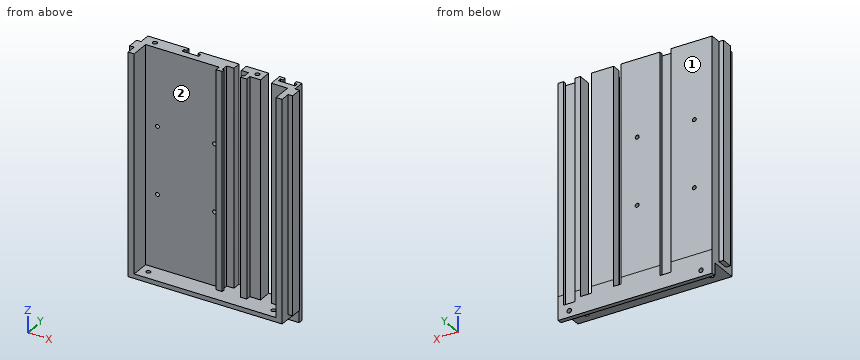
from build123d import *

# Parameters (mm, degrees)
CROQUIS1_W              = 170
CROQUIS1_H              = 50
SALIENTE_EXTRUIR1_DEPTH = 4
CROQUIS3_W              = 20
CROQUIS3_H              = 12.01
SALIENTE_EXTRUIR2_DEPTH = 194
CROQUIS22_W             = 170
CROQUIS22_H             = 21.26
CORTAR_EXTRUIR12_DEPTH  = 10
CROQUIS23_W             = 170
CROQUIS23_H             = 8.12284292
SALIENTE_EXTRUIR6_DEPTH = 11
CROQUIS25_W             = 6.514763964
CROQUIS25_H             = 194
CORTAR_EXTRUIR16_DEPTH  = 10
CROQUIS27_R             = 1.75
CORTAR_EXTRUIR17_DEPTH  = 30.74
CORTAR_EXTRUIR18_DEPTH  = 197
CROQUIS29_W             = 31.946298055
CROQUIS29_H             = 28.740140904
CORTAR_EXTRUIR19_DEPTH  = 197
CROQUIS30_R             = 2
CORTAR_EXTRUIR20_DEPTH  = 197
CROQUIS31_R             = 2
UNI_N_TECHO_DEPTH       = 10
CROQUIS33_R             = 2
CORTAR_EXTRUIR22_DEPTH  = 10
CROQUIS35_W             = 138.053701945
CROQUIS35_H             = 11
CORTAR_EXTRUIR24_DEPTH  = 4.12
SALIENTE_EXTRUIR7_DEPTH = 194


with BuildPart() as part:
    # Croquis1 → Saliente-Extruir1 (new body)
    with BuildSketch(Plane.XY):
        Rectangle(CROQUIS1_W, CROQUIS1_H)
    extrude(amount=SALIENTE_EXTRUIR1_DEPTH)

    # Croquis3 → Saliente-Extruir2 (add)
    with BuildSketch(Plane.XY.offset(4)):
        Polygon((-13.772145946, -12.69105844), (-9.772145946, -12.69105844), (-8.272145946, -12.69105844), (-8.272145946, -9.69105844), (-9.772145946, -9.69105844), (-9.772145946, -3.69105844), (9.772145946, -3.69105844), (9.772145946, -9.69105844), (8.272145946, -9.69105844), (8.272145946, -12.69105844), (9.772145946, -12.69105844), (13.772145946, -12.69105844), (13.772145946, -8.269859096), (23.357191672, -8.269859096), (23.357191672, 3.740140904), (-85, 3.740140904), (-85, -8.269859096), (-13.772145946, -8.269859096), align=None)
        with Locations((43.053701945, -2.264859096)):
            Rectangle(CROQUIS3_W, CROQUIS3_H)
    extrude(amount=SALIENTE_EXTRUIR2_DEPTH)

    # Croquis22 → Cortar-Extruir12 (cut)
    with BuildSketch(Plane(origin=(0, 0, 0), x_dir=(-1, 0, 0), z_dir=(0, 0, -1))):
        with Locations((0, 14.37)):
            Rectangle(CROQUIS22_W, CROQUIS22_H)
    extrude(amount=-CORTAR_EXTRUIR12_DEPTH, mode=Mode.SUBTRACT)

    # Croquis23 → Saliente-Extruir6 (add)
    with BuildSketch(Plane(origin=(0, 0, 0), x_dir=(-1, 0, 0), z_dir=(0, 0, -1))):
        with Locations((0, -0.32142146)):
            Rectangle(CROQUIS23_W, CROQUIS23_H)
    extrude(amount=SALIENTE_EXTRUIR6_DEPTH)

    # Croquis25 → Cortar-Extruir16 (cut)
    with BuildSketch(Plane.XZ.offset(3.69105844)):
        with Locations((0, 101)):
            Rectangle(CROQUIS25_W, CROQUIS25_H)
    extrude(amount=-CORTAR_EXTRUIR16_DEPTH, mode=Mode.SUBTRACT)

    # Croquis27 → Cortar-Extruir17 (cut)
    with BuildSketch(Plane.XZ.offset(8.269859096)):
        with Locations(Location((-69.012145946, 129.117553519, 0), (0, 0, 270))):
            Circle(CROQUIS27_R)
        with Locations(Location((-17.772145946, 129.117553519, 0), (0, 0, 270))):
            Circle(CROQUIS27_R)
        with Locations(Location((-69.012145946, 69.117553519, 0), (0, 0, 270))):
            Circle(CROQUIS27_R)
        with Locations(Location((-17.772145946, 69.117553519, 0), (0, 0, 270))):
            Circle(CROQUIS27_R)
    extrude(amount=-CORTAR_EXTRUIR17_DEPTH, mode=Mode.SUBTRACT)

    # Croquis28 → Cortar-Extruir18 (cut)
    with BuildSketch(Plane.XY.offset(198)):
        Polygon((50.605, 0.740140904), (50.605, -2.259859096), (35.605, -2.259859096), (35.605, 0.740140904), (38.105, 0.740140904), (38.105, 3.740140904), (48.105, 3.740140904), (48.105, 0.740140904), align=None)
        Polygon((-38.105, 3.740140904), (-48.105, 3.740140904), (-48.105, 0.740140904), (-50.605, 0.740140904), (-50.605, -2.259859096), (-35.605, -2.259859096), (-35.605, 0.740140904), (-38.105, 0.740140904), align=None)
    extrude(amount=-CORTAR_EXTRUIR18_DEPTH, mode=Mode.SUBTRACT)

    # Croquis29 → Cortar-Extruir19 (cut)
    with BuildSketch(Plane.XY.offset(4)):
        with Locations((69.026850973, -10.629929548)):
            Rectangle(CROQUIS29_W, CROQUIS29_H)
    extrude(amount=-CORTAR_EXTRUIR19_DEPTH, mode=Mode.SUBTRACT)

    # Croquis30 → Cortar-Extruir20 (cut)
    with BuildSketch(Plane.XY.offset(4)):
        with Locations((-72, -16.634929548)):
            Circle(CROQUIS30_R)
        with Locations((40.053701945, -16.634929548)):
            Circle(CROQUIS30_R)
    extrude(amount=-CORTAR_EXTRUIR20_DEPTH, mode=Mode.SUBTRACT)

    # Croquis31 → Unión techo (cut)
    with BuildSketch(Plane.XY.offset(198)):
        with Locations((-75, -2.264859096)):
            Circle(CROQUIS31_R)
        with Locations((16.857191672, -2.264859096)):
            Circle(CROQUIS31_R)
    extrude(amount=-UNI_N_TECHO_DEPTH, mode=Mode.SUBTRACT)

    # Croquis33 → Cortar-Extruir22 (cut)
    with BuildSketch(Plane.XZ.offset(4.38284292)):
        with Locations(Location((-75, -5.5, 0), (0, 0, 270))):
            Circle(CROQUIS33_R)
        with Locations(Location((43.053701945, -5.5, 0), (0, 0, 270))):
            Circle(CROQUIS33_R)
    extrude(amount=-CORTAR_EXTRUIR22_DEPTH, mode=Mode.SUBTRACT)

    # Croquis35 → Cortar-Extruir24 (cut)
    with BuildSketch(Plane.XZ.offset(4.38284292)):
        with Locations((-15.973149027, -5.5)):
            Rectangle(CROQUIS35_W, CROQUIS35_H)
    extrude(amount=-CORTAR_EXTRUIR24_DEPTH, mode=Mode.SUBTRACT)

    # Croquis36 → Saliente-Extruir7 (add)
    with BuildSketch(Plane.XY.offset(4)):
        Polygon((-85, -8.269859096), (-79.581388396, -8.269859096), (-79.581388396, -25), (-85, -25), (-85, -16.259859096), (-89, -16.259859096), (-89, -6.259859096), (-85, -6.259859096), align=None)
        Polygon((53.053701945, -8.269859096), (53.053701945, -6.259859096), (57.053701945, -6.259859096), (57.053701945, -16.259859096), (53.053701945, -16.259859096), (53.053701945, -25), (47.63509034, -25), (47.63509034, -8.269859096), align=None)
    extrude(amount=SALIENTE_EXTRUIR7_DEPTH)


solid = part.part
Check sheet for the modelled part. Datum: model origin and axes. Units: mm. Face numbers are marked on the shaded views. Round coordinates to 2 decimals unless told otherwise and drop trailing zeros. Order: outer loops, then holes, each group sorted by start corner. A loop starts at its lowest first (then second) coordinate and runs counter-clockwise, first axis right, second up.
(1) Draft check along X on the marked faces 1 and 2. Enter one of: pulls with the +X half, pulls with the -X half, needs draft (parallel to the pull), parting line crosses it, or undercut.
(2) Go/stop test with flat-tipped pins: P1, Ø6, axis at y = 0.5, z = 103.5, coming from the +X side; P2, Ø2, axis at x = -5.5, z = 119.5, coming from the -Y side; P3, Ø2, axis at x = 36.5, z = 145.5, coming from the -Y side. Record where each tip stops, or that it passes through.
(3) Scan lines: probe 1 along X at (y, z) = (0.25, 80.5) (3 decimals); probe 2 along X at (y, z) = (-11.5, 115); probe 3 along X at (y, z) = (-4, 157.5). Record each from-to range of solid material in increasing order.
(4) Cross-section at A-A, the plane x = -45. Enter the section's corners in (y, z), and give its area (3 significant figures).
(5) Cross-section at C-C, the plane y = -21.25. Enter the section's corners in (x, z), and give its area (3 significant figures).
(6) Cross-section at B-B, the plane z = 50. State how many separate pieces and enclosed holes the cut face has, and give its area (3 significant figures).
Check sheet entries:
1. face 1: needs draft
1. face 2: undercut
2. P1: stops at x = 53.05
2. P2: stops at y = -3.69
2. P3: stops at y = -8.27
3. probe 1: x = -85 to -50.605, -35.605 to -3.257, 3.257 to 23.357, 33.054 to 35.605, 50.605 to 53.054
3. probe 2: x = -89 to -79.58, -13.77 to -8.27, 8.27 to 13.77, 47.64 to 57.05
3. probe 3: x = -85 to -9.77, 9.77 to 23.36, 33.05 to 53.05
4. outline: (-25, 0) - (-0.26, 0) - (-0.26, -11) - (3.74, -11) - (3.74, 1) - (-2.26, 1) - (-2.26, 198) - (-8.27, 198) - (-8.27, 4) - (-25, 4) - close
4. area: 1,310 mm2
5. outline: (-85, 0) - (53.05, 0) - (53.05, 198) - (47.64, 198) - (47.64, 4) - (-79.58, 4) - (-79.58, 198) - (-85, 198) - close
5. area: 2,650 mm2
6. separate pieces: 3
6. enclosed holes: 0
6. area: 1,560 mm2
